Geometry check sheet. Reference: the model listing, model coordinates, mm. Face numbers are marked on the shaded views. Coordinates: 2 decimals unless noted, no trailing zeros. Loops run counter-clockwise (first coordinate to the right, second up) from the corner with the lowest first, then second, coordinate; pieces in that order, holes last.
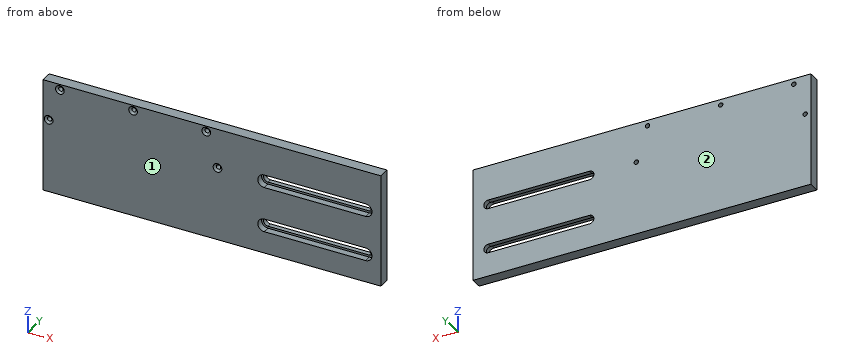
from build123d import *

# Parameters (mm, degrees)
SKETCH2_W                                          = 381
SKETCH2_H                                          = 127
BOSS_EXTRUDE1_DEPTH                                = 12.7
CUT_EXTRUDE1_DEPTH                                 = 12.7
CSK_FOR_10_FLAT_HEAD_MACHINE_SCREW_100_D           = 4.9784
CSK_FOR_10_FLAT_HEAD_MACHINE_SCREW_100_CSINK_D     = 9.779
CSK_FOR_10_FLAT_HEAD_MACHINE_SCREW_100_CSINK_ANGLE = 100
CSK_FOR_10_FLAT_HEAD_MACHINE_SCREW_2_D             = 4.9784
CSK_FOR_10_FLAT_HEAD_MACHINE_SCREW_2_CSINK_D       = 9.779
CSK_FOR_10_FLAT_HEAD_MACHINE_SCREW_2_CSINK_ANGLE   = 100
CUT_EXTRUDE3_DEPTH                                 = 7.62


with BuildPart() as part:
    # Sketch2 → Boss-Extrude1 (new body)
    with BuildSketch(Plane(origin=(0, 0, 0), x_dir=(1, 0, 0), z_dir=(0, 1, 0))):
        Rectangle(SKETCH2_W, SKETCH2_H)
    extrude(amount=BOSS_EXTRUDE1_DEPTH)

    # Sketch8 → Cut-Extrude1 (cut)
    with BuildSketch(Plane.XZ):
        with BuildLine():
            Line((59.055, 23.9776), (173.355, 23.9776))
            ThreePointArc((173.355, 23.9776), (178.2826, 19.05), (173.355, 14.1224))
            Line((173.355, 14.1224), (59.055, 14.1224))
            ThreePointArc((59.055, 14.1224), (54.1274, 19.05), (59.055, 23.9776))
        make_face()
        with BuildLine():
            Line((59.055, -26.8224), (173.355, -26.8224))
            ThreePointArc((173.355, -26.8224), (178.2826, -31.75), (173.355, -36.6776))
            Line((173.355, -36.6776), (59.055, -36.6776))
            ThreePointArc((59.055, -36.6776), (54.1274, -31.75), (59.055, -26.8224))
        make_face()
    extrude(amount=-CUT_EXTRUDE1_DEPTH, mode=Mode.SUBTRACT)

    # CSK for _10 Flat Head Machine Screw _100 (through all)
    with Locations(Plane(origin=(0, 0, 0), x_dir=(-1, 0, 0), z_dir=(0, -1, 0))):
        with Locations((171.45, -57.15), (88.9, -57.15), (6.35, -57.15)):
            CounterSinkHole(CSK_FOR_10_FLAT_HEAD_MACHINE_SCREW_100_D / 2, CSK_FOR_10_FLAT_HEAD_MACHINE_SCREW_100_CSINK_D / 2, counter_sink_angle=CSK_FOR_10_FLAT_HEAD_MACHINE_SCREW_100_CSINK_ANGLE)

    # CSK for _10 Flat Head Machine Screw  2 (through all)
    with Locations(Plane(origin=(0, 0, 0), x_dir=(-1, 0, 0), z_dir=(0, -1, 0))):
        with Locations((184.15, -19.05), (-6.35, -19.05)):
            CounterSinkHole(CSK_FOR_10_FLAT_HEAD_MACHINE_SCREW_2_D / 2, CSK_FOR_10_FLAT_HEAD_MACHINE_SCREW_2_CSINK_D / 2, counter_sink_angle=CSK_FOR_10_FLAT_HEAD_MACHINE_SCREW_2_CSINK_ANGLE)

    # Sketch16 → Cut-Extrude3 (cut)
    with BuildSketch(Plane.XZ):
        with BuildLine():
            Line((59.055, 26.289), (173.355, 26.289))
            ThreePointArc((173.355, 26.289), (180.594, 19.05), (173.355, 11.811))
            Line((173.355, 11.811), (59.055, 11.811))
            ThreePointArc((59.055, 11.811), (51.816, 19.05), (59.055, 26.289))
        make_face()
        with BuildLine():
            Line((59.055, -24.511), (173.355, -24.511))
            ThreePointArc((173.355, -24.511), (180.594, -31.75), (173.355, -38.989))
            Line((173.355, -38.989), (59.055, -38.989))
            ThreePointArc((59.055, -38.989), (51.816, -31.75), (59.055, -24.511))
        make_face()
    extrude(amount=-CUT_EXTRUDE3_DEPTH, mode=Mode.SUBTRACT)


solid = part.part
(1) Sectioned sample at A-A on y = 10.5. Record the cut outline in (x, z) (3 decimals).
Findings:
outline: (-190.5, -63.5) - (190.5, -63.5) - (190.5, 63.5) - (-190.5, 63.5) - close; hole circle Ø4.978 at (-184.15, 19.05); hole circle Ø4.978 at (-171.45, 57.15); hole circle Ø4.978 at (-88.9, 57.15); hole circle Ø4.978 at (-6.35, 57.15); hole circle Ø4.978 at (6.35, 19.05); hole (59.055, -36.678) - (173.355, -36.678) arc R4.928 ccw to (173.355, -26.822) - (59.055, -26.822) arc R4.928 ccw to start; hole (59.055, 14.122) - (173.355, 14.122) arc R4.928 ccw to (173.355, 23.978) - (59.055, 23.978) arc R4.928 ccw to start
(2) Scan lines: L1, parallel to Z at x = 155, y = 9; L2, parallel to Z at x = 128, y = 7.5; L3, parallel to X at y = 8.75, z = 57.15. Record each from-to range of solid material in increasing order.
Findings:
L1: z = -63.5 to -36.68, -26.82 to 14.12, 23.98 to 63.5
L2: z = -63.5 to -38.99, -24.51 to 11.81, 26.29 to 63.5
L3: x = -190.5 to -173.94, -168.96 to -91.39, -86.41 to -8.84, -3.86 to 190.5
(3) Gauge pin test, flat end, axial feed: pin 1 Ø11.5 at (x, z) = (148.5, -30.5) entering from -Y. Record the tip position at first contact, or that the pin passes through.
Findings:
pin 1: stops at y = 7.62
(4) Draft check along Y on the marked faces 1 and 2. Enter one of: +Y half, -Y half, draft (parallel to the pull), parting line (faces both ways), or undercut.
Findings:
face 1: -Y half
face 2: +Y half
